Autodesk Inventor part; units mm, degrees
ref_plane "YZ Plane" through (0, 0, 0) normal (1, 0, 0) x (0, 1, 0)
ref_plane "XZ Plane" through (0, 0, 0) normal (0, 1, 0) x (-1, 0, 0)
ref_plane "XY Plane" through (0, 0, 0) normal (0, 0, 1) x (1, 0, 0)
sketch "Sketch1" plane through (0, 0, 0) normal (0, 1, 0) x (-1, 0, 0)
  line L0 (-3.175, -3.175) -> (3.175, -3.175)
  line L1 (3.175, -3.175) -> (3.175, 3.175)
  line L2 (3.175, 3.175) -> (-3.175, 3.175)
  line L3 (-3.175, 3.175) -> (-3.175, -3.175)
  line L4 (-3.175, -3.175) -> (3.175, 3.175) construction
  line L5 (3.175, -3.175) -> (-3.175, 3.175) construction
  point P0 (0, 0)
  dimension "d0" = 6.35
  dimension "d1" = 6.35
extrude "Extrusion1" add sketch "Sketch1" along normal blind 86.36
fillet "Fillet1" radius 1.5875 4 edges at (3.175, 43.18, 3.175) (3.175, 43.18, -3.175) (-3.175, 43.18, -3.175) (-3.175, 43.18, 3.175)
fillet "Fillet2" radius 0.7937 16 edges at (2.71, 0, -2.71) (0, 0, -3.175) (-2.71, 0, -2.71) (-3.175, 0, 0) (-2.71, 0, 2.71) (0, 0, 3.175) (2.71, 0, 2.71) (3.175, 0, 0) (2.71, 86.36, -2.71) (0, 86.36, -3.175) (-2.71, 86.36, -2.71) (-3.175, 86.36, 0) (-2.71, 86.36, 2.71) (0, 86.36, 3.175) (2.71, 86.36, 2.71) (3.175, 86.36, 0)
sketch "Sketch2" plane through (3.175, 0.7937, 1.5875) normal (1, 0, 0) x (0, 0, -1)
  circle A0 centre (1.5875, 2.3813) radius 1.9844
  line L0 (0, -0.7937) -> (3.175, -0.7937)
  point P0 (1.5875, -0.7937)
  dimension "d6" = 3.9688
  dimension "d7" = 3.175
extrude "Extrusion2" cut sketch "Sketch2" against normal blind 88.9
sketch "Sketch3" plane through (3.175, 85.5662, 1.5875) normal (1, 0, 0) x (0, 0, -1)
  arc A0 (3.175, -81.2006) -> (0, -81.2006) centre (1.5875, -82.3912) ccw
  circle A1 centre (1.5875, -32.785) radius 1.9844
  point P0 (1.5875, -85.5662)
  dimension "d10" = 3.9688
  dimension "d11" = 49.6062
extrude "Extrusion3" cut sketch "Sketch3" against normal blind 88.9
properties part number "wedgeb" material "Stainless Steel"
Input: part model. Units: mm. Frame: model coordinates. Give positions to 0.01 mm unless a question says otherwise; leave off trailing zeros. Order: outer loops, then holes, each group sorted by start corner. A loop starts at its lowest first (then second) coordinate and runs counter-clockwise, first axis right, second up. Notation, with made-up numbers: (38, 44.25) - (55, 44.25) arc R16 ccw to (55, 48.25) - close; hole circle Ø8 at (-34, -38.5). An arc over 180 degrees is marked (long way). Answer as a JSON object with one key per item and string values. Group by question number.
Q1. Line query: probe 1 along Y at (x, z) = (-0.5, 0.25); probe 2 along Y at (x, z) = (2.5, 0.5); probe 3 along Z at (x, y) = (1.75, 33). Output: solid intervals per line, ascending.
Q2. Cut plane A-A, the plane z = 0. Output: boundary loops of the cut face in (x, y) (3 decimals).
Q3. Cut plane C-C, the plane y = 70.5. Output: boundary loops of the cut face in (x, z) (1 decimal), then the cut area to 3 significant figures.
Q4. Mould query, pull axis Y, two halves, no side actions, for faces 1 (the face through (3.175, 28, 0)), 2 (the face through (0.044, 50.844, 0.43)), 3 (the face through (0.044, 1.238, 0.43)), 4 (the face through (0, 0, 0)). Classes: pulls with the +Y half, pulls with the -Y half, needs draft (parallel to the pull), parting line crosses it, or undercut.
Q5. Cut plane B-B, the plane x = 0.5. Output: boundary loops of the cut face in (y, z) (3 decimals).
Results:
{
 "1": {"probe 1": "0 to 1.21, 5.14 to 50.81, 54.75 to 86.36", "probe 2": "0.01 to 1.25, 5.1 to 50.86, 54.7 to 86.35", "probe 3": "-3.17 to 3.17"},
 "2": {"outline": "(-3.175, 0.794) arc R0.794 ccw to (-2.381, 0) - (2.381, 0) arc R0.794 ccw to (3.175, 0.794) - (3.175, 1.191) - (-3.175, 1.191) - close; (-3.175, 5.159) - (3.175, 5.159) - (3.175, 50.797) - (-3.175, 50.797) - close; (-3.175, 54.766) - (3.175, 54.766) - (3.175, 85.566) arc R0.794 ccw to (2.381, 86.36) - (-2.381, 86.36) arc R0.794 ccw to (-3.175, 85.566) - close"},
 "3": {"outline": "(-3.2, -1.6) arc R1.6 ccw to (-1.6, -3.2) - (1.6, -3.2) arc R1.6 ccw to (3.2, -1.6) - (3.2, 1.6) arc R1.6 ccw to (1.6, 3.2) - (-1.6, 3.2) arc R1.6 ccw to (-3.2, 1.6) - close", "area": "38.2 mm^2"},
 "4": {"face 1": "needs draft", "face 2": "undercut", "face 3": "undercut", "face 4": "pulls with the -Y half"},
 "5": {"outline": "(0, -2.381) arc R0.794 ccw to (0.794, -3.175) - (85.566, -3.175) arc R0.794 ccw to (86.36, -2.381) - (86.36, 2.381) arc R0.794 ccw to (85.566, 3.175) - (0.794, 3.175) arc R0.794 ccw to (0, 2.381) - close; hole circle Ø3.969 at (3.175, 0); hole circle Ø3.969 at (52.781, 0)"}
}
